Check sheet for the modelled part. Datum: model origin and axes. Units: mm. Give positions to 0.01 mm unless a question says otherwise; leave off trailing zeros. Loops run counter-clockwise (first coordinate to the right, second up) from the corner with the lowest first, then second, coordinate; pieces in that order, holes last. Notation, with made-up numbers: M 45.25,82 L 59.25,82 A12 ccw 59.25,93 Z; hole C -28,81 d5. An arc over 180 degrees is marked long. Use one line per item in the form item = value.
from build123d import *

# Parameters (mm, degrees)
F1_DEPTH = 2
F2_R     = 5
F4_D     = 20
F4_DEPTH = 50
F4_TIP   = 6.0086061903


with BuildPart() as f1:
    # F0 (on Top) → F1 (new body)
    with BuildSketch(Plane.XY):
        Polygon((-300, 100), (-300, -100), (-100, -100), (-100, -300), (100, -300), (100, -100), (300, -100), (300, 100), (100, 100), (100, 300), (-100, 300), (-100, 100), align=None)
    extrude(amount=F1_DEPTH)

    # F2
    f2_edges = [f1.edges().sort_by_distance(p)[0] for p in [
        (-300, -100, 1),
        (-100, -100, 1),
        (-100, -300, 1),
        (100, -300, 1),
        (-300, 100, 1),
        (-100, 300, 1),
        (100, 300, 1),
        (100, 100, 1),
        (300, 100, 1),
        (300, -100, 1),
        (-100, 100, 1),
        (100, -100, 1),
    ]]
    fillet(f2_edges, radius=F2_R)

    # F4
    with Locations(Plane(origin=(0, 0, 0), x_dir=(1, 0, 0), z_dir=(0, 0, -1))):
        with Locations((-276.0063111782, -68.7044858932), (-47.2173690796, -51.3386949897), (77.8317674994, 65.5974373221), (-36.1162610352, 260.7022225857), (211.3765329123, -65.6183883548), (30.6354723871, -259.6825659275)):
            Hole(F4_D / 2, depth=F4_DEPTH)
            with Locations((0, 0, -(F4_DEPTH + F4_TIP / 2))):  # 118° drill point
                Cone(0, F4_D / 2, F4_TIP, mode=Mode.SUBTRACT)


solid = f1.part
1) Section check B-B (x = -116). Record the cut outline in (y, z), then the cut area to 3 significant figures.
Evaluation:
outline = M -100,0 L 100,0 L 100,2 L -100,2 Z
area = 400 mm^2
2) Scan lines: line 1 (X direction, y = 71.5, z = 1.7) (3 decimals); line 2 (X direction, y = -164, z = 1.55). Record each from-to range of solid material in increasing order.
Evaluation:
line_1 = -300 to -285.608, -266.405 to 203.289, 219.464 to 300
line_2 = -100 to 100
3) Section check A-A (z = 1.1). State how many separate pieces and enclosed holes the cut face has, then the cut area to 3 significant figures.
Evaluation:
separate_pieces = 1
enclosed_holes = 6
area = 198,000 mm^2
4) Release check for a two-part mould opening along Y. For faces 1 (the face through (-4, 4, 0)), 2 (the face through (72.46, -74.03, 1.01)) record: pulls with the +Y half, pulls with the -Y half, needs draft (parallel to the pull), parting line crosses it, or undercut.
Evaluation:
face_1 = needs draft
face_2 = undercut
5) Depth check by flat-ended pin: pin 1 Ø1 at (y, z) = (237.5, 1) entering from +X; pin 2 Ø0.6 at (x, z) = (213.5, 1) entering from +Y. Enter the tip coordinate at first touch or a pass-through.
Evaluation:
pin_1 = 100
pin_2 = 100
